Geometry check sheet. Reference: the model listing, model coordinates, mm. A direction names the side the tool comes from. Coordinates: 2 decimals unless noted, no trailing zeros. Write each loop counter-clockwise with the first axis right and the second up, starting at its lowest first coordinate (ties: lowest second). Pieces come first, ordered by that corner, then holes. Notation, with made-up numbers: (79.25, -22) -> (120.25, -22) arc R17 ccw to (120.25, 4) -> close; hole circle Ø7 at (78.5, 77). An arc over 180 degrees is marked (long way). Answer in a Markdown table with one row per item. Add a question column.
1. Cross-section at C-C on y = -3.5. Record the cut outline in (x, z), and give its area (3 significant figures).
2. Mould release check, pull along X, two halves, no side actions. Record for faces 1 (the flat face through (-10, 0, 2)), 2 (the cylindrical face through (7.641, 4.365, 0.887)), 3 (the flat face through (-2, 5, 0)): pulls with the +X half, pulls with the -X half, needs draft (parallel to the pull), parting line crosses it, or undercut.
3. Cross-section at B-B on z = 0.95. Record the cut outline in (x, y) (3 decimals).
4. Set-up check for faces 4 (the flat face through (10, 0, 2)), 5 (the cylindrical face through (6.77, 3.44, 0.89)), 6 (the flat face through (-3.55, -2, 2.88)): record each of +Z, -Z, +X, -X, +Y, -Y from which the full face is reachable in a straight line by a thin tool's end or side.
5. Scan lines: L1, parallel to X at y = 0.75, z = 1.3; L2, parallel to Y at x = -0.75, z = 3.55; L3, parallel to Y at x = 1.5, z = 3.65. Record each from-to range of solid material in increasing order. Write a range as from..to.
6. Cross-section at A-A on x = -1. Record the cut outline in (y, z).
7. Cross-section at D-D on z = 3.2. Record the cut outline in (x, y) (3 decimals), and give its area (3 significant figures).
```python
from build123d import *

# Parameters (mm, degrees)
PAD_DEPTH            = 18
SKETCH002_R          = 0.75
PAD001_DEPTH         = 1.8
CYLINDER_R           = 5.025
CYLINDER_DEPTH       = 1.8
BODY_PLACEMENT_ANGLE = 60
BOX_W                = 20
BOX_H                = 20
BOX_DEPTH            = 4


with BuildPart() as motorbody:
    # Sketch001 → Pad (new body)
    with BuildSketch(Plane.XY):
        with BuildLine():
            ThreePointArc((-2.940238, 4.075), (-5.025, 0), (-2.940238, -4.075))
            Line((-2.940238, -4.075), (2.940238, -4.075))
            ThreePointArc((2.940238, -4.075), (5.025, 0), (2.940238, 4.075))
            Line((-2.940238, 4.075), (2.940238, 4.075))
        make_face()
    extrude(amount=PAD_DEPTH)

    # Sketch002 → Pad001 (join)
    with BuildSketch(Plane.XY):
        with BuildLine():
            ThreePointArc((1.85, 6.95), (0, 8.8), (-1.85, 6.95))
            Line((-1.85, 6.95), (-1.85, -6.950003))
            ThreePointArc((-1.85, -6.950003), (2e-06, -8.8), (1.85, -6.949999))
            Line((1.85, 6.95), (1.85, -6.949999))
        make_face()
        with Locations((0, 6.95)):
            Circle(SKETCH002_R, mode=Mode.SUBTRACT)
        with Locations((0, -6.95)):
            Circle(SKETCH002_R, mode=Mode.SUBTRACT)
    extrude(amount=PAD001_DEPTH)

    # Cylinder → Cylinder (join)
    with BuildSketch(Plane.XY):
        Circle(CYLINDER_R)
    extrude(amount=CYLINDER_DEPTH)


with BuildPart() as motorbody_1:
    # Body placement: moved
    add(motorbody.part.rotate(Axis((0, 0, 0), (0, 0, -1)), BODY_PLACEMENT_ANGLE))


with BuildPart() as motortestholder:
    # Box → Box (new body)
    with BuildSketch(Plane(origin=(-10, -10, 0), x_dir=(1, 0, 0), z_dir=(0, 0, 1))):
        with Locations((10, 10)):
            Rectangle(BOX_W, BOX_H)
    extrude(amount=BOX_DEPTH)

    # Cut: cut MotorBody
    add(motorbody_1.part, mode=Mode.SUBTRACT)


solid = motortestholder.part
```
Results found:
| question | item | result |
|---|---|---|
| 1 | outline | (-10, 0) -> (-7.87, 0) -> (-7.87, 1.8) -> (-6.77, 1.8) -> (-6.77, 0) -> (-5.27, 0) -> (-5.27, 1.8) -> (-2.68, 1.8) -> (-2.68, 4) -> (-10, 4) -> close; (3.61, 0) -> (10, 0) -> (10, 4) -> (3.61, 4) -> close |
| 1 | area | 48.2 mm^2 |
| 2 | face 1 | pulls with the -X half |
| 2 | face 2 | undercut |
| 2 | face 3 | needs draft |
| 3 | outline | (-10, -10) -> (10, -10) -> (10, 10) -> (-10, 10) -> close; circle Ø1.5 at (-6.019, -3.475); circle Ø1.5 at (6.019, 3.475); hole (-6.944, -1.873) arc R1.85 ccw to (-5.094, -5.077) -> (-3.121, -3.938) arc R5.025 ccw to (4.971, 0.734) -> (6.944, 1.873) arc R1.85 ccw to (5.094, 5.077) -> (3.121, 3.938) arc R5.025 ccw to (-4.971, -0.734) -> close |
| 4 | face 4 | +Z, -Z, +X, +Y, -Y |
| 4 | face 5 | -Z |
| 4 | face 6 | +Z, -Z |
| 5 | L1 | x = -10..-4.97, 5..10 |
| 5 | L2 | y = -10..-4.97, 4.97..10 |
| 5 | L3 | y = -10..-4.8, 4.8..10 |
| 6 | outline | (-10, 0) -> (-4.92, 0) -> (-4.92, 4) -> (-10, 4) -> close; (4.92, 0) -> (10, 0) -> (10, 4) -> (4.92, 4) -> close |
| 7 | outline | (-10, -10) -> (10, -10) -> (10, 10) -> (-10, 10) -> close; hole (-4.999, 0.509) -> (-2.059, -4.584) arc R5.025 ccw to (4.999, -0.509) -> (2.059, 4.584) arc R5.025 ccw to start |
| 7 | area | 328 mm^2 |
